from build123d import *

# Parameters (mm, degrees)
SKETCH1_W           = 22
SKETCH1_H           = 10
BOSS_EXTRUDE1_DEPTH = 6
SKETCH2_W           = 10
SKETCH2_H           = 10
BOSS_EXTRUDE2_DEPTH = 12
SKETCH3_R           = 1.75
CUT_EXTRUDE1_DEPTH  = 31.133038347
CUT_EXTRUDE2_DEPTH  = 3


with BuildPart() as part:
    # Sketch1 → Boss-Extrude1 (new body)
    with BuildSketch(Plane(origin=(0, 0, 0), x_dir=(1, 0, 0), z_dir=(0, 1, 0))):
        with Locations((11, 5)):
            Rectangle(SKETCH1_W, SKETCH1_H)
    extrude(amount=BOSS_EXTRUDE1_DEPTH)

    # Sketch2 → Boss-Extrude2 (add)
    with BuildSketch(Plane(origin=(0, 6, 0), x_dir=(1, 0, 0), z_dir=(0, 1, 0))):
        with Locations((5, 5)):
            Rectangle(SKETCH2_W, SKETCH2_H)
    extrude(amount=BOSS_EXTRUDE2_DEPTH)

    # Sketch3 → Cut-Extrude1 (cut, through all)
    with BuildSketch(Plane(origin=(0, 18, 0), x_dir=(1, 0, 0), z_dir=(0, 1, 0))):
        with Locations(Location((5, 5, 0), (0, 0, 270))):
            Circle(SKETCH3_R)
    extrude(amount=-CUT_EXTRUDE1_DEPTH, mode=Mode.SUBTRACT)

    # Sketch4 → Cut-Extrude2 (cut)
    with BuildSketch(Plane.XZ):
        Polygon((1.824573519, -5), (3.41228676, -7.75), (6.58771324, -7.75), (8.175426481, -5), (6.58771324, -2.25), (3.41228676, -2.25), align=None)
    extrude(amount=-CUT_EXTRUDE2_DEPTH, mode=Mode.SUBTRACT)


solid = part.part
Can you work these out from the model? Positions are in its coordinate system, mm. A direction names the side the tool comes from. Coordinates: 2 decimals unless noted, no trailing zeros. Order: outer loops, then holes, each group sorted by start corner. A loop starts at its lowest first (then second) coordinate and runs counter-clockwise, first axis right, second up. Notation, with made-up numbers: (53.5, -0.5) - (94.5, -0.5) arc R14 ccw to (94.5, 24.5) - close; hole circle Ø3 at (7, 25.5). An arc over 180 degrees is marked (long way). Answer as a JSON object with one key per item and string values. Group by question number.
Q1. Imagine slicing it at D-D (x = 2.25). Please give me the cut outline in (y, z), and give its area (3 significant figures).
Q2. Imagine slicing it at B-B (y = 1.5). Please give me the cut outline in (x, z).
Q3. We'd pull the mould along X, two halves only. Please class faces 1 (the face through (0, 9, -5)), 2 (the face through (11, 0, -5)), 3 (the face through (3.29, 10.6, -5.38)): +X half, -X half, draft (parallel to the pull), parting line (faces both ways), or undercut.
Q4. Imagine slicing it at A-A (x = 5). Please give me the cut outline in (y, z).
Q5. Will these pins go through, and if not, where does the flat tip stop? P1, Ø3, axis at y = 11.5, z = -6, coming from the +X side; P2, Ø3, axis at x = 14.5, y = 8.5, coming from the -Z side; P3, Ø5, axis at x = 16, z = -3, coming from the +Y side; P4, Ø8, axis at x = 7.5, y = 12, coming from the +Z side.
Q6. I need wall thicknesses on line 1 (X direction, y = 7.25, z = -5); line 2 (Z direction, x = 6, y = 1); line 3 (Y direction, x = 20.5, z = -7.25). Which ranges of each line are inside material? Lowest first, please. Write a range as from..to.
Q7. On a 3-axis mill with a long thin cutter (end or side, diameter ignored), from which of +Z, -Z, +X, -X, +Y, -Y can I reach the whole of each face in a straight line? I mean faces 4 (the face through (7, 18, -5)), 5 (the face through (10, 12, -5)), 6 (the face through (2.61, 1.48, -6.36)). Say none if no direction works.
Q8. Imagine slicing it at C-C (y = 12). Please give me the cut outline in (x, z), and give its area (3 significant figures).
Determined:
{
 "1": {"outline": "(0, -10) - (18, -10) - (18, 0) - (0, 0) - (0, -4.26) - (3, -4.26) - (3, -5.74) - (0, -5.74) - close", "area": "176 mm2"},
 "2": {"outline": "(0, -10) - (22, -10) - (22, 0) - (0, 0) - close; hole (1.82, -5) - (3.41, -7.75) - (6.59, -7.75) - (8.18, -5) - (6.59, -2.25) - (3.41, -2.25) - close"},
 "3": {"face 1": "-X half", "face 2": "draft", "face 3": "undercut"},
 "4": {"outline": "(0, -10) - (18, -10) - (18, -6.75) - (3, -6.75) - (3, -7.75) - (0, -7.75) - close; (0, -2.25) - (3, -2.25) - (3, -3.25) - (18, -3.25) - (18, 0) - (0, 0) - close"},
 "5": {"P1": "stops at x = 10", "P2": "passes through", "P3": "stops at y = 6", "P4": "stops at z = 0"},
 "6": {"line 1": "x = 0..3.25, 6.75..10", "line 2": "z = -10..-7.75, -2.25..0", "line 3": "y = 0..6"},
 "7": {"face 4": "+Z, -Z, +X, -X, +Y", "face 5": "+Z, -Z, +X, +Y", "face 6": "-Y"},
 "8": {"outline": "(0, -10) - (10, -10) - (10, 0) - (0, 0) - close; hole circle Ø3.5 at (5, -5)", "area": "90.4 mm2"}
}
